Design review of the part built by this model. Coordinates are the model's own, in mm. A direction names the side the tool comes from. Round coordinates to 2 decimals unless told otherwise and drop trailing zeros. Loops run counter-clockwise (first coordinate to the right, second up) from the corner with the lowest first, then second, coordinate; pieces in that order, holes last. Notation, with made-up numbers: M 57,44.5 L 112,44.5 A24 cw 112,81.5 Z; hole C 12,78.25 d2. An arc over 180 degrees is marked long. Use a Markdown table: item, result.
from build123d import *

# Parameters (mm, degrees)
F0_R     = 9.525
F0_R_2   = 3.175
F1_DEPTH = 25.4
F2_W     = 5.595942471
F2_H     = 0.8117107314
F4_W     = 5.7437195435
F4_H     = 10.4512684047
F4_H_2   = 14.192732051
F4_W_2   = 5.8874822214
F4_H_3   = 10.6966430321
F5_DEPTH = 6.985
F6_R     = 1.016


with BuildPart() as f1:
    # F0 (on Top) → F1 (new body)
    with BuildSketch(Plane.XY):
        Circle(F0_R)
        Circle(F0_R_2, mode=Mode.SUBTRACT)
    extrude(amount=-F1_DEPTH)

    # F2 (on Front) → F3 (revolve, cut)
    with BuildSketch(Plane.XZ):
        with BuildLine():
            Line((11.056942471, -4.953), (5.461, -4.953))
            ThreePointArc((5.461, -4.953), (7.5418947367, -7.9335299315), (11.056942471, -7.0071817232))
            Line((11.056942471, -7.0071817232), (11.056942471, -4.953))
        make_face()
        with BuildLine():
            ThreePointArc((11.056942471, -7.0071817232), (11.6165299315, -6.0471052633), (11.811, -4.953))
            ThreePointArc((11.811, -4.953), (8.636, -1.778), (5.461, -4.953))
            Line((5.461, -4.953), (11.056942471, -4.953))
            Line((11.056942471, -4.953), (11.056942471, -7.0071817232))
        make_face()
        Polygon((5.461, -9.9557107314), (5.461, -9.144), (0, -9.144), (0, -34.544), (12.0641607791, -34.544), (12.0641607791, -9.144), (11.056942471, -9.144), (11.056942471, -9.9557107314), align=None)
        with BuildLine():
            ThreePointArc((11.056942471, -7.0071817232), (7.5418947367, -7.9335299315), (5.461, -4.953))
            Line((5.461, -4.953), (5.461, -9.144))
            Line((5.461, -9.144), (11.056942471, -9.144))
            Line((11.056942471, -9.144), (11.056942471, -7.0071817232))
        make_face()
        with Locations((8.2589712355, -9.5498553657)):
            Rectangle(F2_W, F2_H)
    revolve(axis=Axis((0, 0, -25.4), (0, 0, 1)), mode=Mode.SUBTRACT)

    # F4 (on face) → F5 (cut)
    with BuildSketch(Plane(origin=(0, 0, -9.144), x_dir=(1, 0, 0), z_dir=(0, 0, -1))):
        with Locations((-8.3328597717, -5.2256342024)):
            Rectangle(F4_W, F4_H)
        with Locations((-8.3328597717, 7.0963660255)):
            Rectangle(F4_W, F4_H_2)
        with Locations((8.4047411107, 5.3483215161)):
            Rectangle(F4_W_2, F4_H_3)
        Polygon((11.3484822214, 0), (5.461, 0), (5.461, -9.0715084225), (5.461, -9.423006326), (11.6024822214, -9.423006326), (11.6024822214, 0), align=None)
        with BuildLine():
            Line((-5.08, -2.0040261974), (-5.08, 2.0040261974))
            ThreePointArc((-5.08, 2.0040261974), (-5.3649045192, 1.0199610287), (-5.461, 0))
            ThreePointArc((-5.461, 0), (-5.3649045192, -1.0199610287), (-5.08, -2.0040261974))
        make_face()
        with BuildLine():
            ThreePointArc((-5.461, 0), (-5.3649045192, 1.0199610287), (-5.08, 2.0040261974))
            Line((-5.08, 2.0040261974), (-5.08, 14.192732051))
            Line((-5.08, 14.192732051), (-5.461, 14.192732051))
            Line((-5.461, 14.192732051), (-5.461, 0))
        make_face()
        with BuildLine():
            Line((-5.08, -11.2700536847), (-5.08, -2.0040261974))
            ThreePointArc((-5.08, -2.0040261974), (-5.3649045192, -1.0199610287), (-5.461, 0))
            Line((-5.461, 0), (-5.461, -10.4512684047))
            Line((-5.461, -10.4512684047), (-5.461, -11.2700536847))
            Line((-5.461, -11.2700536847), (-5.08, -11.2700536847))
        make_face()
        with BuildLine():
            Line((5.461, -9.0715084225), (5.461, 0))
            ThreePointArc((5.461, 0), (5.3649045192, -1.0199610287), (5.08, -2.0040261974))
            Line((5.08, -2.0040261974), (5.08, -9.0715084225))
            Line((5.08, -9.0715084225), (5.461, -9.0715084225))
        make_face()
        with BuildLine():
            ThreePointArc((5.08, -2.0040261974), (5.3649045192, -1.0199610287), (5.461, 0))
            ThreePointArc((5.461, 0), (5.3649045192, 1.0199610287), (5.08, 2.0040261974))
            Line((5.08, 2.0040261974), (5.08, -2.0040261974))
        make_face()
        with BuildLine():
            ThreePointArc((5.08, 2.0040261974), (5.3649045192, 1.0199610287), (5.461, 0))
            Line((5.461, 0), (5.461, 10.6966430321))
            Line((5.461, 10.6966430321), (5.08, 10.6966430321))
            Line((5.08, 10.6966430321), (5.08, 2.0040261974))
        make_face()
    extrude(amount=-F5_DEPTH, mode=Mode.SUBTRACT)

    # F6
    f6_edges = [f1.edges().sort_by_distance(p)[0] for p in [
        (5.08, 0, -2.159),
        (-5.08, 0, -2.159),
    ]]
    fillet(f6_edges, radius=F6_R)


solid = f1.part
1. Take a section at A-A on y = 0. Give the boundary of the cut face in (x, z) (3 decimals), and give its area (3 significant figures).
Check values:
| item | result |
|---|---|
| outline | M -9.525,-1.905 A3.175 cw -7.128,-2.159 L -6.096,-2.159 A1.016 cw -5.08,-3.175 L -5.08,-9.144 L -3.175,-9.144 L -3.175,0 L -9.525,0 Z; M 3.175,-9.144 L 5.08,-9.144 L 5.08,-3.175 A1.016 cw 6.096,-2.159 L 7.128,-2.159 A3.175 cw 9.525,-1.905 L 9.525,0 L 3.175,0 Z |
| area | 53.1 mm² |
2. The part is to be moulded in two halves that separate along X. For faces 5 (the face through (5.08, 0, -6)), 6 (the face through (-0.69, -3.1, -4.51)), 7 (the face through (-5.08, 0, -6)), say which applies: pulls with the +X half, pulls with the -X half, needs draft (parallel to the pull), parting line crosses it, or undercut.
Check values:
| item | result |
|---|---|
| face 5 | pulls with the +X half |
| face 6 | undercut |
| face 7 | pulls with the -X half |
3. Wall thickness on line 1 along Y through (x, z) = (0, -5.25) (3 decimals); line 2 along Z through (x, y) = (-6.25, -3); line 3 along X through (y, z) = (2.25, -3): over which ranges is each line inside the solid? List them lowest first. Write a range as from..to.
Check values:
| item | result |
|---|---|
| line 1 | y = -5.461..-3.175, 3.175..5.461 |
| line 2 | z = -2.16..0 |
| line 3 | x = -5.1..-2.24, 2.24..5.1 |
4. Insertion check: pin 1 (1 mm diameter, centred on x = 0.5, y = -6.5, fed in from -Z); pin 2 (1.1 mm diameter, centred on x = -6.5, y = -1, fed in from -Z); pin 3 (1.8 mm diameter, centred on y = 0.5, z = -5.5, fed in from +X). Each pin has a flat end and moves straight along its axis. Give the tip position at first contact, or say it passes through.
Check values:
| item | result |
|---|---|
| pin 1 | stops at z = -3.15 |
| pin 2 | stops at z = -2.17 |
| pin 3 | stops at x = 5.08 |
5. Take a section at B-B on x = 0. Give the boundary of the cut face in (y, z) (3 decimals).
Check values:
| item | result |
|---|---|
| outline | M -9.525,-1.905 A3.175 cw -5.461,-4.953 L -5.461,-9.144 L -3.175,-9.144 L -3.175,0 L -9.525,0 Z; M 3.175,-9.144 L 5.461,-9.144 L 5.461,-4.953 A3.175 cw 9.525,-1.905 L 9.525,0 L 3.175,0 Z |
6. Take a section at D-D on z = -1. Give the boundary of the cut face in (x, y) (3 decimals).
Check values:
| item | result |
|---|---|
| outline | C 0,0 d19.05; hole C 0,0 d6.35 |
7. Machinability: for faces 1 (the face through (6.5, -0.1, -2.159)), 2 (the face through (-6.5, -0.1, -2.159)), 3 (the face through (-0.09, -5.46, -7.08)), 4 (the face through (0.09, 5.46, -7.08)), which of the approach directions +Z, -Z, +X, -X, +Y, -Y give a long, thin tool a straight path to every point of the face, cutting with its end or side? Answer none if there is none.
Check values:
| item | result |
|---|---|
| face 1 | -Z, +X, +Y, -Y |
| face 2 | -Z, -X, +Y, -Y |
| face 3 | -Z, -Y |
| face 4 | -Z, +Y |
8. Take a section at C-C on z = -6.25. Give the boundary of the cut face in (x, y) (3 decimals).
Check values:
| item | result |
|---|---|
| outline | M -5.08,-2.004 A5.461 ccw 5.08,-2.004 L 5.08,2.004 A5.461 ccw -5.08,2.004 Z; hole C 0,0 d6.35 |
